Check sheet for the modelled part. Datum: model origin and axes. Units: mm. Face numbers are marked on the shaded views. A direction names the side the tool comes from. Coordinates: 2 decimals unless noted, no trailing zeros. Loops run counter-clockwise (first coordinate to the right, second up) from the corner with the lowest first, then second, coordinate; pieces in that order, holes last. Notation, with made-up numbers: M 32,71.25 L 67,71.25 A5 ccw 67,80.25 Z; hole C 62.5,-1 d9. An arc over 180 degrees is marked long. Write each question's results on one line, items separated by ' | '. Start each with the question number.
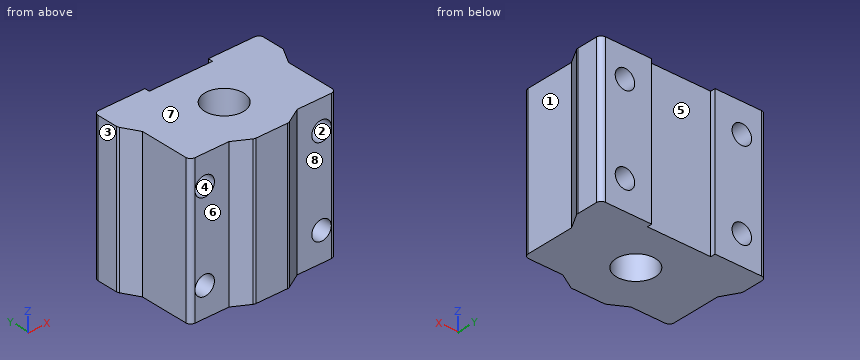
from build123d import *

# Parameters (mm, degrees)
BOSS_EXTRUDE1_DEPTH = 30
FILLET1_R           = 1
CUT_EXTRUDE1_REACH  = 42.902
SKETCH2_R           = 4
CUT_EXTRUDE2_REACH  = 42.902
SKETCH3_R           = 2
SKETCH4_W           = 13
SKETCH4_H           = 30
CUT_EXTRUDE3_DEPTH  = 1


with BuildPart() as part:
    # Sketch1 → Boss-Extrude1 (new body)
    with BuildSketch(Plane.XY):
        Polygon((-17, 0), (17, 0), (17, -5.5), (15, -9), (15, -20), (7, -20), (3.5, -22), (-3.5, -22), (-7, -20), (-15, -20), (-15, -9), (-17, -5.5), align=None)
    extrude(amount=BOSS_EXTRUDE1_DEPTH)

    # Fillet1
    fillet1_edges = [part.edges().sort_by_distance(p)[0] for p in [
        (-17, 0, 15),
        (17, 0, 15),
        (17, -5.5, 15),
        (15, -20, 15),
        (3.5, -22, 15),
        (-3.5, -22, 15),
        (-15, -20, 15),
        (-17, -5.5, 15),
    ]]
    fillet(fillet1_edges, radius=FILLET1_R)

    # Sketch2 → Cut-Extrude1 (cut, up to next)
    with BuildSketch(Plane.XY.offset(30), mode=Mode.PRIVATE) as cut_extrude1_sk1:
        with Locations((0, -11)):
            Circle(SKETCH2_R)
    cut_extrude1_tool1 = extrude(cut_extrude1_sk1.sketch, amount=-CUT_EXTRUDE1_REACH, mode=Mode.PRIVATE) & part.part
    add(cut_extrude1_tool1.solids().sort_by_distance((0, -11, 30))[0], mode=Mode.SUBTRACT)

    # Sketch3 → Cut-Extrude2 (cut, up to next)
    with BuildSketch(Plane(origin=(0, 0, 0), x_dir=(1, 0, 0), z_dir=(0, 1, 0)), mode=Mode.PRIVATE) as cut_extrude2_sk1:
        with Locations(Location((-12, -6, 0), (0, 0, 180))):
            Circle(SKETCH3_R)
    cut_extrude2_tool1 = extrude(cut_extrude2_sk1.sketch, amount=-CUT_EXTRUDE2_REACH, mode=Mode.PRIVATE) & part.part
    # Sketch3 → Cut-Extrude2 (cut, up to next)
    with BuildSketch(Plane(origin=(0, 0, 0), x_dir=(1, 0, 0), z_dir=(0, 1, 0)), mode=Mode.PRIVATE) as cut_extrude2_sk2:
        with Locations(Location((-12, -24, 0), (0, 0, 180))):
            Circle(SKETCH3_R)
    cut_extrude2_tool2 = extrude(cut_extrude2_sk2.sketch, amount=-CUT_EXTRUDE2_REACH, mode=Mode.PRIVATE) & part.part
    # Sketch3 → Cut-Extrude2 (cut, up to next)
    with BuildSketch(Plane(origin=(0, 0, 0), x_dir=(1, 0, 0), z_dir=(0, 1, 0)), mode=Mode.PRIVATE) as cut_extrude2_sk3:
        with Locations(Location((12, -24, 0), (0, 0, 180))):
            Circle(SKETCH3_R)
    cut_extrude2_tool3 = extrude(cut_extrude2_sk3.sketch, amount=-CUT_EXTRUDE2_REACH, mode=Mode.PRIVATE) & part.part
    # Sketch3 → Cut-Extrude2 (cut, up to next)
    with BuildSketch(Plane(origin=(0, 0, 0), x_dir=(1, 0, 0), z_dir=(0, 1, 0)), mode=Mode.PRIVATE) as cut_extrude2_sk4:
        with Locations(Location((12, -6, 0), (0, 0, 180))):
            Circle(SKETCH3_R)
    cut_extrude2_tool4 = extrude(cut_extrude2_sk4.sketch, amount=-CUT_EXTRUDE2_REACH, mode=Mode.PRIVATE) & part.part
    add(cut_extrude2_tool1.solids().sort_by_distance((-12, 0, 6))[0], mode=Mode.SUBTRACT)
    add(cut_extrude2_tool2.solids().sort_by_distance((-12, 0, 24))[0], mode=Mode.SUBTRACT)
    add(cut_extrude2_tool3.solids().sort_by_distance((12, 0, 24))[0], mode=Mode.SUBTRACT)
    add(cut_extrude2_tool4.solids().sort_by_distance((12, 0, 6))[0], mode=Mode.SUBTRACT)

    # Sketch4 → Cut-Extrude3 (cut)
    with BuildSketch(Plane(origin=(0, 0, 0), x_dir=(1, 0, 0), z_dir=(0, 1, 0))):
        with Locations((0, -15)):
            Rectangle(SKETCH4_W, SKETCH4_H)
    extrude(amount=-CUT_EXTRUDE3_DEPTH, mode=Mode.SUBTRACT)


solid = part.part
Item 1: Section check D-D (x = -12). Record the cut outline in (y, z), plus the area to 3 significant figures.
Item 2: Section check A-A (y = -11). Record the cut outline in (x, z).
Item 3: Thickness scan on line 1 (Z direction, x = 12, y = -11); line 2 (Y direction, x = 0, z = 15); line 3 (X direction, y = -11.75, z = 4.75). Record the ranges inside material, lowest first.
Item 4: Depth check by flat-ended pin: P1, Ø8, axis at y = -9.5, z = 14, coming from the +X side; P2, Ø1, axis at x = 5, y = -18.5, coming from the -Z side; P3, Ø5, axis at x = -12, z = 24, coming from the -Y side; P4, Ø5, axis at y = -15.5, z = 19, coming from the +X side. Enter the tip coordinate at first touch or a pass-through.
Item 5: Tool access check on the marked faces 4, 5, 6, 7 and 8. Record the directions out of +Z, -Z, +X, -X, +Y, -Y that give a thin tool (end or side, any length) a straight path to the whole face; none if there is none.
Item 6: Section check B-B (x = 0). Record the cut outline in (y, z).
Item 7: Section check C-C (z = 15.5). Record the cut outline in (x, y), plus the area to 3 significant figures.
Item 8: Release check for a two-part mould opening along X. For the marked faces 1, 2 and 3 record: +X half, -X half, draft (parallel to the pull), parting line (faces both ways), or undercut.
Computed values:
1) outline: M -20,0 L 0,0 L 0,4 L -20,4 Z; M -20,8 L 0,8 L 0,22 L -20,22 Z; M -20,26 L 0,26 L 0,30 L -20,30 Z | area: 440 mm²
2) outline: M -15,0 L -4,0 L -4,30 L -15,30 Z; M 4,0 L 15,0 L 15,30 L 4,30 Z; hole C -12,6 d4; hole C -12,24 d4; hole C 12,6 d4; hole C 12,24 d4
3) line 1: z = 0 to 4, 8 to 22, 26 to 30 | line 2: y = -22 to -15, -7 to -1 | line 3: x = -15 to -13.56, -10.44 to -3.93, 3.93 to 10.44, 13.56 to 15
4) P1: stops at x = 16.96 | P2: stops at z = 0 | P3: stops at y = -20 | P4: stops at x = 15
5) face 4: +Y, -Y | face 5: +Z, -Z, +Y | face 6: +Z, -Z, -X, -Y | face 7: +Z, +X, -X, +Y, -Y | face 8: +Z, -Z, +X, -Y
6) outline: M -22,0 L -15,0 L -15,30 L -22,30 Z; M -7,0 L -1,0 L -1,30 L -7,30 Z
7) outline: M -17,-5.23 A1 ccw -16.87,-5.73 L -15,-9 L -15,-19 A1 ccw -14,-20 L -7,-20 L -3.73,-21.87 A1 ccw -3.23,-22 L 3.23,-22 A1 ccw 3.73,-21.87 L 7,-20 L 14,-20 A1 ccw 15,-19 L 15,-9 L 16.87,-5.73 A1 ccw 17,-5.23 L 17,-1 A1 ccw 16,0 L 6.5,0 L 6.5,-1 L -6.5,-1 L -6.5,0 L -16,0 A1 ccw -17,-1 Z; hole C 0,-11 d8 | area: 586 mm²
8) face 1: +X half | face 2: undercut | face 3: -X half
